```python
from build123d import *

# Parameters (mm, degrees)
EXTRUDE1_DEPTH             = 700
SKETCH2_R                  = 1.75
EXTRUDE2_DEPTH             = 6.5
SKETCH_R                   = 3
SKETCH_R_2                 = 1.75
EXTRUDE4_DEPTH             = 3.5
CHAMFER1_SIZE              = 0.2
LPATTERN1_COUNT            = 34
LPATTERN1_PITCH            = 20
CHAMFER1_OF_LPATTERN1_SIZE = 0.2


with BuildPart() as part:
    # Sketch1 → Extrude1 (new body)
    with BuildSketch(Plane.XY):
        with BuildLine():
            Line((-4.3, -3.25), (4.3, -3.25))
            Line((4.3, -3.25), (4.5, -3.05))
            Line((4.5, -3.05), (4.5, 0.455012563))
            ThreePointArc((4.5, 0.455012563), (3.924845827, 0.712323349), (3.617735397, 1.2625))
            Line((3.617735397, 1.2625), (3.15008224, 1.2625))
            Line((3.15008224, 1.2625), (3.15008224, 1.7625))
            Line((3.15008224, 1.7625), (3.65008224, 1.7625))
            ThreePointArc((3.65008224, 1.7625), (3.973877727, 2.229724887), (4.5, 2.444987437))
            Line((4.5, 2.444987437), (4.5, 3.05))
            Line((4.5, 3.05), (4.3, 3.25))
            Line((4.3, 3.25), (-4.3, 3.25))
            Line((-4.3, 3.25), (-4.5, 3.05))
            Line((-4.5, 3.05), (-4.5, 2.444987437))
            ThreePointArc((-4.5, 2.444987437), (-3.973877727, 2.229724887), (-3.65008224, 1.7625))
            Line((-3.65008224, 1.7625), (-3.15008224, 1.7625))
            Line((-3.15008224, 1.7625), (-3.15008224, 1.2625))
            Line((-3.15008224, 1.2625), (-3.617735397, 1.2625))
            ThreePointArc((-3.617735397, 1.2625), (-3.924845827, 0.712323349), (-4.5, 0.455012563))
            Line((-4.5, 0.455012563), (-4.5, -3.05))
            Line((-4.5, -3.05), (-4.3, -3.25))
        make_face()
    extrude(amount=EXTRUDE1_DEPTH)

    # Sketch2 → Extrude2 (cut)
    with BuildSketch(Plane(origin=(0, 3.25, 0), x_dir=(1, 0, 0), z_dir=(0, 1, 0))):
        with Locations((0, -15)):
            Circle(SKETCH2_R)
    extrude2 = extrude(amount=-EXTRUDE2_DEPTH, mode=Mode.SUBTRACT)

    # Sketch → Extrude4 (cut)
    with BuildSketch(Plane(origin=(0, 3.25, 0), x_dir=(1, 0, 0), z_dir=(0, 1, 0))):
        with Locations((0, -15)):
            Circle(SKETCH_R)
        with Locations((0, -15)):
            Circle(SKETCH_R_2, mode=Mode.SUBTRACT)
    extrude4 = extrude(amount=-EXTRUDE4_DEPTH, mode=Mode.SUBTRACT)

    # Chamfer1
    chamfer1_edges = [part.edges().sort_by_distance(p)[0] for p in [
        (-1.75, -3.25, 15),
        (-3, 3.25, 15),
    ]]
    chamfer(chamfer1_edges, length=CHAMFER1_SIZE)

    # LPattern1: Extrude2, Extrude4 ×34
    with Locations(*[(0, 0, i * LPATTERN1_PITCH) for i in range(1, LPATTERN1_COUNT)]):
        add(extrude2, mode=Mode.SUBTRACT)
        add(extrude4, mode=Mode.SUBTRACT)

    # Chamfer1 of LPattern1
    chamfer1_of_lpattern1_edges = [part.edges().sort_by_distance(p)[0] for p in [
        (-1.75, -3.25, 35),
        (-3, 3.25, 35),
        (-1.75, -3.25, 55),
        (-3, 3.25, 55),
        (-1.75, -3.25, 75),
        (-3, 3.25, 75),
        (-1.75, -3.25, 95),
        (-3, 3.25, 95),
        (-1.75, -3.25, 115),
        (-3, 3.25, 115),
        (-1.75, -3.25, 135),
        (-3, 3.25, 135),
        (-1.75, -3.25, 155),
        (-3, 3.25, 155),
        (-1.75, -3.25, 175),
        (-3, 3.25, 175),
        (-1.75, -3.25, 195),
        (-3, 3.25, 195),
        (-1.75, -3.25, 215),
        (-3, 3.25, 215),
        (-1.75, -3.25, 235),
        (-3, 3.25, 235),
        (-1.75, -3.25, 255),
        (-3, 3.25, 255),
        (-1.75, -3.25, 275),
        (-3, 3.25, 275),
        (-1.75, -3.25, 295),
        (-3, 3.25, 295),
        (-1.75, -3.25, 315),
        (-3, 3.25, 315),
        (-1.75, -3.25, 335),
        (-3, 3.25, 335),
        (-1.75, -3.25, 355),
        (-3, 3.25, 355),
        (-1.75, -3.25, 375),
        (-3, 3.25, 375),
        (-1.75, -3.25, 395),
        (-3, 3.25, 395),
        (-1.75, -3.25, 415),
        (-3, 3.25, 415),
        (-1.75, -3.25, 435),
        (-3, 3.25, 435),
        (-1.75, -3.25, 455),
        (-3, 3.25, 455),
        (-1.75, -3.25, 475),
        (-3, 3.25, 475),
        (-1.75, -3.25, 495),
        (-3, 3.25, 495),
        (-1.75, -3.25, 515),
        (-3, 3.25, 515),
        (-1.75, -3.25, 535),
        (-3, 3.25, 535),
        (-1.75, -3.25, 555),
        (-3, 3.25, 555),
        (-1.75, -3.25, 575),
        (-3, 3.25, 575),
        (-1.75, -3.25, 595),
        (-3, 3.25, 595),
        (-1.75, -3.25, 615),
        (-3, 3.25, 615),
        (-1.75, -3.25, 635),
        (-3, 3.25, 635),
        (-1.75, -3.25, 655),
        (-3, 3.25, 655),
        (-1.75, -3.25, 675),
        (-3, 3.25, 675),
    ]]
    chamfer(chamfer1_of_lpattern1_edges, length=CHAMFER1_OF_LPATTERN1_SIZE)


solid = part.part
```
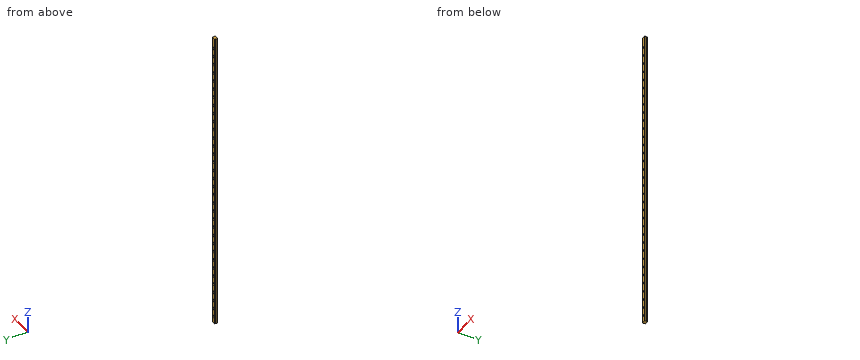
Input: part model. Units: mm. Frame: model coordinates. Give positions to 0.01 mm unless a question says otherwise; leave off trailing zeros. Use a Markdown table: item, result.
Q1. First-contact query: P1, Ø5, axis at x = 0, z = 555, coming from the +Y side; P2, Ø1, axis at x = 3, y = -1.5, coming from the -Z side. Flat tips, straight axial feed; report the tip coordinate or a pass-through.
Entries:
| item | result |
|---|---|
| P1 | stops at y = -0.25 |
| P2 | stops at z = 0 |
Q2. Ray query, probe 1 along X at (y, z) = (1.65, 275); probe 2 along X at (y, z) = (-1.75, 635); probe 3 along Y at (x, z) = (4.25, 638). Return the intervals inside material, ascending. Write a range as from..to.
Entries:
| item | result |
|---|---|
| probe 1 | x = -3.15..-3, 3..3.15 |
| probe 2 | x = -4.5..-1.75, 1.75..4.5 |
| probe 3 | y = -3.25..0.51, 2.39..3.25 |
Q3. Section query A-A, the plane x = 0.25. State how many separate pieces and enclosed holes the cut face has, plus the area to 3 significant figures.
Entries:
| item | result |
|---|---|
| separate pieces | 35 |
| enclosed holes | 0 |
| area | 3,480 mm² |
